Could you check a few things on this drawing? It's one solid part, dimensions in mm from its lowest x, y, z. A direction names the side the tool comes from. Give positions to 0.01 mm unless a question says otherwise; leave off trailing zeros. Write each loop counter-clockwise with the first axis right and the second up, starting at its lowest first coordinate (ties: lowest second). Pieces come first, ordered by that corner, then holes.
1. Suppose I cut it at B-B (z = 12.5). Please give me the cut outline in (x, y), and give its area (3 significant figures).
2. On a 3-axis mill with a long thin cutter (end or side, diameter ignored), from which of +Z, -Z, +X, -X, +Y, -Y can I reach the whole of each face in a straight line? I mean the marked faces 1 and 2. Say none if no direction works.
3. If I drill on probe 1 along Z at (x, y) = (37, 10.75), over which ranges is the centre line in solid material (lowest first)?
4. I'm going to push flat-ended pins straight in: pin 1 (2 mm diameter, centred on x = 32.5, y = 17.5, fed in from +Z); pin 2 (5 mm diameter, centred on x = 11, z = 22.5, fed in from +Y). Where does each tip first touch, or does it pass through?
5. Suppose I cut it at A-A (x = 41). Please give me the cut outline in (y, z), and give its area (3 significant figures).
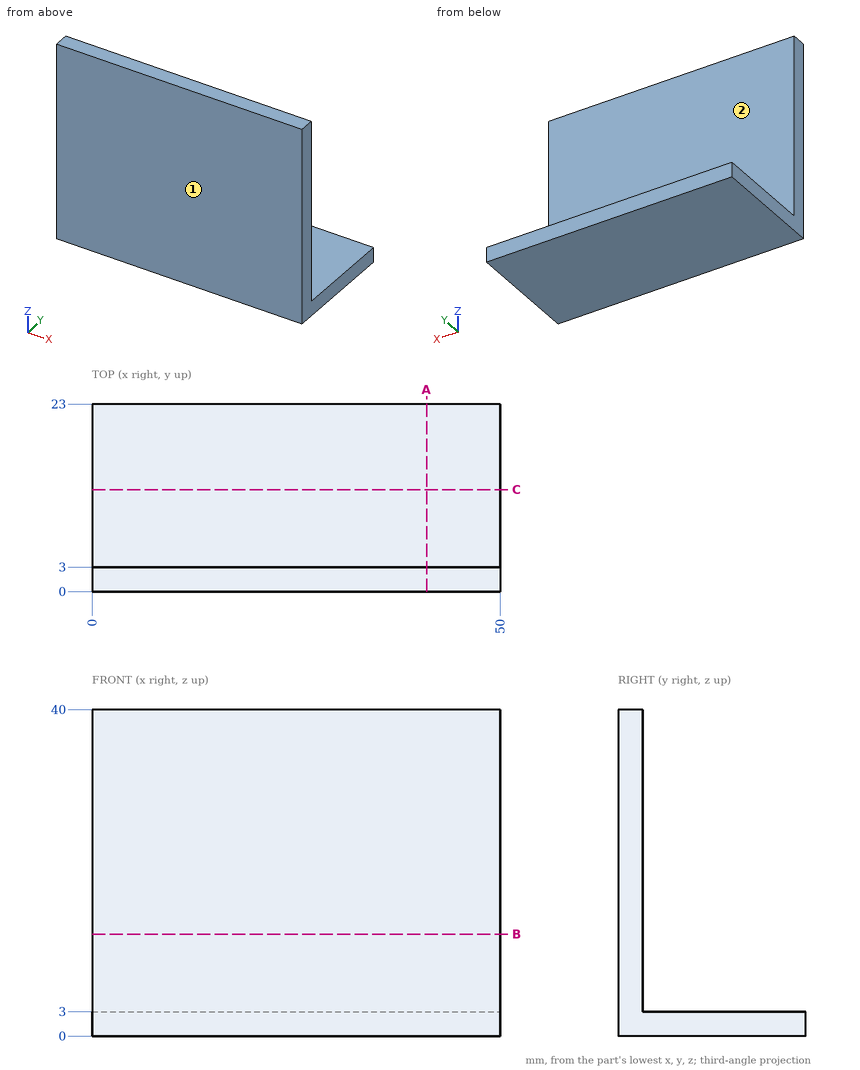
Checks:
1. outline: (0, 0) - (50, 0) - (50, 3) - (0, 3) - close
1. area: 150 mm2
2. face 1: +Z, -Z, +X, -X, -Y
2. face 2: +Z, +X, -X, +Y
3. probe 1: z = 0 to 3
4. pin 1: stops at z = 3
4. pin 2: stops at y = 3
5. outline: (0, 0) - (23, 0) - (23, 3) - (3, 3) - (3, 40) - (0, 40) - close
5. area: 180 mm2
